from build123d import *

# Parameters (mm, degrees)
BOSS_EXTRUDE1_DEPTH   = 2.7686
BOSS_EXTRUDE2_START   = -2.7686
BOSS_EXTRUDE2_DEPTH   = 50.8
BOSS_EXTRUDE2_2_DEPTH = 50.8
SKETCH4_W             = 2.7686
SKETCH4_H             = 50.8
BOSS_EXTRUDE3_DEPTH   = 25.4
CUT_EXTRUDE1_DEPTH    = 47.2186
BOSS_EXTRUDE6_DEPTH   = 44.45


with BuildPart() as part:
    # Sketch1 → Boss-Extrude1 (new body)
    with BuildSketch(Plane(origin=(0, 0, 0), x_dir=(1, 0, 0), z_dir=(0, 1, 0))):
        Polygon((0, 0), (44.45, 0), (172.085, -107.098481425), (-127.635, -107.098481425), align=None)
    extrude(amount=BOSS_EXTRUDE1_DEPTH)



with BuildPart() as body_2:
    # Sketch2 → Boss-Extrude2 (new body)
    with BuildSketch(Plane(origin=(0, 2.7686, 0), x_dir=(1, 0, 0), z_dir=(0, 1, 0)).offset(BOSS_EXTRUDE2_START)):
        Polygon((0, 0), (-127.635, -107.098481425), (-130.4036, -107.098481425), (-2.7686, 0), align=None)
    extrude(amount=BOSS_EXTRUDE2_DEPTH)


with BuildPart() as body_3:
    # Sketch2 → Boss-Extrude2 2 (new body)
    with BuildSketch(Plane(origin=(0, 2.7686, 0), x_dir=(1, 0, 0), z_dir=(0, 1, 0)).offset(BOSS_EXTRUDE2_START)):
        Polygon((44.45, 0), (47.2186, 0), (174.8536, -107.098481425), (172.085, -107.098481425), align=None)
    extrude(amount=BOSS_EXTRUDE2_2_DEPTH)


with BuildPart() as part_1:
    add(part.part)

    add(body_3.part)  # Boss-Extrude3 merges body 3
    # Sketch4 → Boss-Extrude3 (add)
    with BuildSketch(Plane(origin=(0, 0, 0), x_dir=(-1, 0, 0), z_dir=(0, 0, -1))):
        with Locations((-45.8343, 25.4)):
            Rectangle(SKETCH4_W, SKETCH4_H)
    boss_extrude3 = extrude(amount=BOSS_EXTRUDE3_DEPTH)

    # Sketch5 → Cut-Extrude1 (cut)
    with BuildSketch(Plane(origin=(47.2186, 0, 0), x_dir=(0, 0, -1), z_dir=(1, 0, 0))):
        Polygon((17.186035514, 6.697089394), (0, 0), (25.4, 0), (25.4, 14.244871038), (25.4, 50.8), (0, 50.8), align=None)
    cut_extrude1 = extrude(amount=-CUT_EXTRUDE1_DEPTH, mode=Mode.SUBTRACT)


    add(body_2.part)  # Boss-Extrude6 merges body 2
    # Sketch10 → Boss-Extrude6 (add)
    with BuildSketch(Plane.ZY.offset(-44.45)):
        with BuildLine():
            Line((-17.186035514, 6.697089394), (-15.298135688, 8.75161917))
            ThreePointArc((-15.298135688, 8.75161917), (-8.213243481, 4.317554379), (0, 2.7686))
            Line((0, 2.7686), (0, 0))
            Line((0, 0), (-17.186035514, 6.697089394))
        make_face()
    extrude(amount=BOSS_EXTRUDE6_DEPTH)

    # Mirror1: Boss-Extrude3 across plane
    add(boss_extrude3.mirror(Plane.ZY.offset(-22.225)))

    # Mirror2: Cut-Extrude1 across plane
    add(cut_extrude1.mirror(Plane.ZY.offset(-22.225)), mode=Mode.SUBTRACT)


solid = part_1.part
Can you work these out from the model? Positions are in its coordinate system, mm. A direction names the side the tool comes from. Round coordinates to 2 decimals unless told otherwise and drop trailing zeros. Write each loop counter-clockwise with the first axis right and the second up, starting at its lowest first coordinate (ties: lowest second). Pieces come first, ordered by that corner, then holes. Notation, with made-up numbers: M 7.25,32.5 L 39.25,32.5 A25 cw 39.25,58.5 Z; hole C 44,48 d2. An arc over 180 degrees is marked long. Use CSV: the item, a comma, the result in double quotes.
(1) Imagine slicing it at D-D (y = 15). Write out the boundary of the cut face in (x, z) (3 decimals), plus the area to 3 significant figures.
Check values:
outline,"M -130.404,107.098 L -2.769,0 L -2.769,-13.951 L 0,-13.951 L 0,0 L -127.635,107.098 Z; M 44.45,-13.951 L 47.219,-13.951 L 47.219,0 L 174.854,107.098 L 172.085,107.098 L 44.45,0 Z"
area,"670 mm^2"
(2) Imagine slicing it at A-A (y = 27.5). Write out the boundary of the cut face in (x, z) (3 decimals), plus the area to 3 significant figures.
Check values:
outline,"M -130.404,107.098 L -2.769,0 L -2.769,-9.08 L 0,-9.08 L 0,0 L -127.635,107.098 Z; M 44.45,-9.08 L 47.219,-9.08 L 47.219,0 L 174.854,107.098 L 172.085,107.098 L 44.45,0 Z"
area,"643 mm^2"
(3) On a 3-axis mill with a long thin cutter (end or side, diameter ignored), from which of +Z, -Z, +X, -X, +Y, -Y can I reach the whole of each face in a straight line? I mean faces 1 (the flat face through (45.85, 29.06, -8.47)), 2 (the flat face through (-2.769, 19, -5)), 3 (the flat face through (20, 0, 66)), 4 (the flat face through (47.219, 19, -5)), 5 (the cylindrical face through (22.54, 4.36, -8.32)). Say none if no direction works.
Check values:
face 1,"-Z, +X, -X, +Y"
face 2,"-Z, -X, +Y, -Y"
face 3,"+Z, -Z, +X, -X, -Y"
face 4,"-Z, +X, +Y, -Y"
face 5,"+Z, +Y"
(4) I need wall thicknesses on line 1 along X through (y, z) = (36, -3); line 2 along Y through (x, z) = (15, 11.5); line 3 along X through (y, z) = (16.5, 21.5). Which ranges of each line are inside material? Lowest first, please.
Check values:
line 1,"-2.77 to 0, 44.45 to 47.22"
line 2,"0 to 2.77"
line 3,"-28.39 to -25.62, 70.07 to 72.84"
(5) Imagine slicing it at C-C (z = 62.5). Write out the boundary of the cut face in (x, y), plus the area to 3 significant figures.
Check values:
outline,"M -77.25,0 L 121.7,0 L 121.7,50.8 L 118.93,50.8 L 118.93,2.77 L -74.48,2.77 L -74.48,50.8 L -77.25,50.8 Z"
area,"817 mm^2"
(6) Imagine slicing it at B-B (x = 21). Write out the boundary of the cut face in (y, z).
Check values:
outline,"M 0,0 L 6.7,-17.19 L 8.75,-15.3 A22.55 cw 2.77,0 L 2.77,107.1 L 0,107.1 Z"
(7) I'm going to push flat-ended pins straight in: pin 1 (1.5 mm diameter, centred on x = 86, y = 8.5, fed in from +Z); pin 2 (12 mm diameter, centred on x = 22.5, y = 13, fed in from +Z); pin 3 (2 mm diameter, centred on x = -31, z = 20.5, fed in from -Y); pin 4 (12 mm diameter, centred on x = 113, y = 43, fed in from -Z). Where does each tip first touch, or does it pass through?
Check values:
pin 1,"z = 35.49"
pin 2,"z = -13.15"
pin 3,"through"
pin 4,"z = 50.16"
